Autodesk Inventor part; units mm, degrees
ref_plane "YZ Plane" through (0, 0, 0) normal (1, 0, 0) x (0, 1, 0)
ref_plane "XZ Plane" through (0, 0, 0) normal (0, 1, 0) x (-1, 0, 0)
ref_plane "XY Plane" through (0, 0, 0) normal (0, 0, 1) x (1, 0, 0)
sketch "Sketch1" plane through (0, 0, 0) normal (0, 1, 0) x (-1, 0, 0)
  circle A0 centre (0, 0) radius 1.25
  line L0 (0, 0) -> (2.5, 0) construction
  line L1 (1.4352, -1.4352) -> (2.0297, 0)
  line L2 (1.4352, 1.4352) -> (0, 2.0297)
  line L3 (0, 2.0297) -> (-1.4352, 1.4352)
  line L4 (-1.4352, 1.4352) -> (-2.0297, 0)
  line L5 (-2.0297, 0) -> (-1.4352, -1.4352)
  line L6 (-1.4352, -1.4352) -> (0, -2.0297)
  line L7 (0, -2.0297) -> (1.4352, -1.4352)
  line L8 (2.0297, 0) -> (1.4352, 1.4352)
  dimension "d0" = 2.5
extrude "Extrusion1" add sketch "Sketch1" along normal blind 15.84
properties part number "base_telaio_casters"
Model file for the job. Use its own axes, mm. Give positions to 0.01 mm unless a question says otherwise; leave off trailing zeros. Order: outer loops, then holes, each group sorted by start corner. A loop starts at its lowest first (then second) coordinate and runs counter-clockwise, first axis right, second up. Notation, with made-up numbers: M 22,47.5 L 69,47.5 A22 cw 69,86.5 Z; hole C 59.5,86.25 d3. An arc over 180 degrees is marked long. Put each result on its own line as item: value. Start each with the question number.
(1) Pull direction X, two halves, no side cores. Call faces 1 (the face through (-0.728, 7.809, 1.728)), 2 (the face through (0.708, 7.809, 1.737)), 3 (the face through (0.27, 7.81, 1.22)): released by +X, released by -X, zero draft, split by the parting line, or undercut.
(2) Band-saw the part on D-D on z = 1.7. Give the cut face in (x, y), then the cut area to 3 significant figures.
(3) Drill centre lines: L1, parallel to Z at x = -0.6, y = 1.25; L2, parallel to Z at x = 0.4, y = 11; L3, parallel to X at y = 6.25, z = -0.75. Where is each one in solid material? Low to high. Write a range as [from, to].
(4) Band-saw the part on C-C on z = -1. Give the cut face in (x, y).
(5) Pin check, flat tip, straight feed: pin 1 Ø2 at (x, z) = (0, 0) entering from +Y. Stop position of the tip, or through.
(6) Band-saw the part on B-B on z = 0.8. Give the cut face in (x, y), then the cut area to 3 significant figures.
(7) Band-saw the part on A-A on y = 7.5. Give the cut face in (x, z).
Results below:
1. face 1: released by -X
1. face 2: released by +X
1. face 3: undercut
2. outline: M -0.8,0 L 0.8,0 L 0.8,15.84 L -0.8,15.84 Z
2. area: 25.2 mm2
3. L1: z = [-1.78, -1.1], [1.1, 1.78]
3. L2: z = [-1.86, -1.18], [1.18, 1.86]
3. L3: x = [-1.72, -1], [1, 1.72]
4. outline: M -1.62,0 L -0.75,0 L -0.75,15.84 L -1.62,15.84 Z; M 0.75,0 L 1.62,0 L 1.62,15.84 L 0.75,15.84 Z
5. pin 1: passes through
6. outline: M -1.7,0 L -0.96,0 L -0.96,15.84 L -1.7,15.84 Z; M 0.96,0 L 1.7,0 L 1.7,15.84 L 0.96,15.84 Z
6. area: 23.4 mm2
7. outline: M -2.03,0 L -1.44,-1.44 L 0,-2.03 L 1.44,-1.44 L 2.03,0 L 1.44,1.44 L 0,2.03 L -1.44,1.44 Z; hole C 0,0 d2.5
